Autodesk Inventor part; units mm, degrees
ref_plane "YZ Plane" through (0, 0, 0) normal (1, 0, 0) x (0, 1, 0)
ref_plane "XZ Plane" through (0, 0, 0) normal (0, 1, 0) x (-1, 0, 0)
ref_plane "XY Plane" through (0, 0, 0) normal (0, 0, 1) x (1, 0, 0)
sketch "Sketch3" plane through (0, 0, 0) normal (0, 0, 1) x (1, 0, 0)
  line L0 (0, 0) -> (12.2, 0)
  line L1 (12.2, 0) -> (12.2, -32.5)
  line L2 (12.2, -32.5) -> (0, -32.5)
  line L3 (0, -32.5) -> (0, 0)
  dimension "d11" = 12.2
  dimension "d12" = 32.5
extrude "Extrusion3" add sketch "Sketch3" along normal blind 2.5
sketch "Sketch4" plane through (0, 0, 2.5) normal (0, 0, 1) x (1, 0, 0)
  line L0 (0, 0) -> (0, -32.5)
  line L1 (12.2, -32.5) -> (12.2, 0)
  line L2 (0, -5) -> (12.2, -5)
  line L3 (12.2, -5) -> (12.2, -27.5)
  line L4 (12.2, -27.5) -> (0, -27.5)
  line L5 (0, -27.5) -> (0, -5)
  line L6 (12.2, 0) -> (0, 0)
  dimension "d15" = 22.5
  dimension "d16" = 5
extrude "Extrusion4" add sketch "Sketch4" along normal blind 16.5 contours L2 L1 L4 L0
sketch "Sketch5" plane through (0, 0, 0) normal (0, 0, -1) x (-1, 0, 0)
  line L0 (0, -5) -> (-12.2, -5)
  line L1 (-12.2, -27.5) -> (0, -27.5)
  line L2 (-12.2, -5) -> (0, -5)
  line L3 (0, -5) -> (0, -27.5)
  line L4 (0, -27.5) -> (-12.2, -27.5)
  line L5 (-12.2, -27.5) -> (-12.2, -5)
  point P0 (0, 0)
extrude "Extrusion5" add sketch "Sketch5" along normal blind 4
sketch "Sketch6" plane through (0, 0, 0) normal (0, 0, -1) x (-1, 0, 0)
  circle A0 centre (-6.1, -2.5) radius 1.25
  circle A1 centre (-6.1, -30) radius 1.25
  line L0 (-12.2, -27.5) -> (0, -27.5)
  line L1 (-12.2, 0) -> (0, 0)
  line L2 (-12.2, -5) -> (-12.2, 0)
  line L3 (-12.2, -32.5) -> (-12.2, -27.5)
  dimension "d21" = 2.5
  dimension "d22" = 2.5
  dimension "d23" = 2.5
  dimension "d24" = 2.5
  dimension "d25" = 6.1
  dimension "d26" = 6.1
extrude "Extrusion6" cut sketch "Sketch6" against normal up to surface (2.5 mm away)
sketch "Sketch7" plane through (0, 0, -4) normal (0, 0, -1) x (-1, 0, 0)
  circle A0 centre (-6.1, -11.1) radius 6.1
  line L0 (0, -5) -> (0, -27.5)
  line L1 (0, -5) -> (-12.2, -5)
  circle A1 centre (-6.1, -16.5) radius 2.8
  line L2 (-12.2, -27.5) -> (0, -27.5)
  point P0 (0, 0)
  point P1 (-3.3001, -16.5194)
  point P2 (-8.8999, -16.5194)
  point P3 (-6.1, -5)
  point P4 (0, -11.1)
  dimension "d29" = 6.1
  dimension "d30" = 12.2
  dimension "d33" = 5.6
  dimension "d34" = 11
extrude "Extrusion7" add sketch "Sketch7" along normal blind 4.5 contours A0 A1 | A1 A0 | A0 A1
sketch "Sketch8" plane through (0, 0, -8.5) normal (0, 0, -1) x (-1, 0, 0)
  arc A0 (-6.1, -5) -> (-12.2, -11.1) centre (-6.1, -11.1) ccw
  circle A1 centre (-6.1, -11.1) radius 2.5
  point P0 (0, 0)
  dimension "d35" = 5
extrude "Extrusion8" add sketch "Sketch8" along normal blind 5
properties part number "servo_motor" material "Nylon 6/6"
Could you check a few things on this model? Use its own coordinates, in mm. A direction names the side the tool comes from. Round coordinates to 2 decimals unless told otherwise and drop trailing zeros. Loops run counter-clockwise (first coordinate to the right, second up) from the corner with the lowest first, then second, coordinate; pieces in that order, holes last. Notation, with made-up numbers: M -14.5,58 L 43.5,58 A24 ccw 43.5,83 Z; hole C 14,70 d2. An arc over 180 degrees is marked long. Write item = value, one per line.
1. I want a section at C-C, the plane x = 10. Write out the boundary of the cut face in (y, z), and give its area (3 significant figures).
Results below:
outline = M -32.5,0 L -27.5,0 L -27.5,-4 L -15.79,-4 L -15.79,-8.5 L -6.41,-8.5 L -6.41,-4 L -5,-4 L -5,0 L 0,0 L 0,2.5 L -5,2.5 L -5,19 L -27.5,19 L -27.5,2.5 L -32.5,2.5 Z
area = 585 mm²
2. I want a section at A-A, the plane y = -30. Write out the boundary of the cut face in (x, z), and give its area (4 significant figures).
Results below:
outline = M 0,0 L 4.85,0 L 4.85,2.5 L 0,2.5 Z; M 7.35,0 L 12.2,0 L 12.2,2.5 L 7.35,2.5 Z
area = 24.25 mm²
3. I need wall thicknesses on probe 1 along Y at (x, z) = (6.1, 1.5); probe 2 along Z at (x, y) = (5.25, -26.5); probe 3 along Z at (x, y) = (11.5, -29.5). Which ranges of each line are inside material? Lowest first, please.
Results below:
probe_1 = -32.5 to -31.25, -28.75 to -3.75, -1.25 to 0
probe_2 = -4 to 19
probe_3 = 0 to 2.5
4. Will these pins go through, and if not, where does the flat tip stop? P1, Ø6, axis at x = 9, z = 10.5, coming from the -Y side; P2, Ø3, axis at x = 6.1, y = -30, coming from the +Z side; P3, Ø2, axis at x = 5.5, z = -2, coming from the +Y side; P4, Ø2, axis at x = 6.1, y = -2.5, coming from the +Z side.
Results below:
P1 = -27.5
P2 = 2.5
P3 = -5
P4 = through
5. I want a section at D-D, the plane y = -18. Write out the boundary of the cut face in (x, z), and give its area (3 significant figures).
Results below:
outline = M 0,-4 L 3.74,-4 L 3.74,-8.5 L 8.46,-8.5 L 8.46,-4 L 12.2,-4 L 12.2,19 L 0,19 Z
area = 302 mm²
6. I want a section at B-B, the plane z = 11.5. Write out the boundary of the cut face in (x, y).
Results below:
outline = M 0,-27.5 L 12.2,-27.5 L 12.2,-5 L 0,-5 Z
7. Which directions (+Z, -Z, +X, -X, +Y, -Y) give clear straight access to the entire face, cutting with the end or side of a thin tool? Please do faces 1 (the face through (6, -27.5, -2)), 2 (the face through (6, -5, -2)), 3 (the face through (11, -6, -4)).
Results below:
face_1 = -Z, +X, -X, -Y
face_2 = -Z, +X, -X, +Y
face_3 = -Z, +X, +Y
